Verification items for the finished model (mm, model axes). Face numbers are marked on the shaded views. Round coordinates to 2 decimals unless told otherwise and drop trailing zeros. Write each loop counter-clockwise with the first axis right and the second up, starting at its lowest first coordinate (ties: lowest second). Pieces come first, ordered by that corner, then holes. Notation, with made-up numbers: M 3,-31 L 23,-31 A23 cw 23,8 Z; hole C 22,21.5 d1. An arc over 180 degrees is marked long. One line per question, with ' | ' between items. Start each with the question number.
Q1. Cross-section at A-A (y = 0). Record the boundary of the cut face in (x, z), then the cut area to 3 significant figures.
Q2. Release check for a two-part mould opening along Y. For the marked faces 1, 2 and 3 record: released by +Y, released by -Y, zero draft, split by the parting line, or undercut.
Q3. Thickness scan on line 1 along X through (y, z) = (40.5, 35); line 2 along Y through (x, z) = (-33.5, 27.5); line 3 along Y through (x, z) = (-32.5, 31). Record the ranges inside material, lowest first. Write a range as from..to.
Q4. Cross-section at D-D (x = 40). Record the boundary of the cut face in (y, z), then the cut area to 3 significant figures.
Q5. Gauge pin test, flat ends, axial feed: pin 1 (5 mm diameter, centred on x = 40.5, z = 32.5, fed in from +Y); pin 2 (10 mm diameter, centred on y = 19.5, z = 19.5, fed in from -X); pin 3 (3 mm diameter, centred on x = 9, y = -47.5, fed in from +Z); pin 4 (6 mm diameter, centred on y = -35.5, z = 6.5, fed in from +X). Record the tip position at first contact, or that the pin passes through.
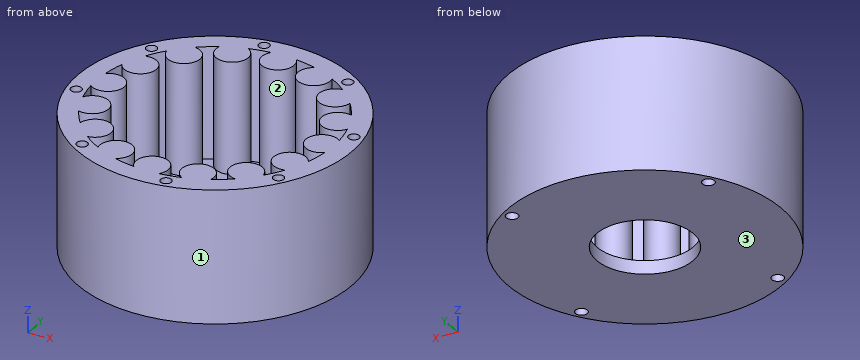
from build123d import *

# Parameters (mm, degrees)
SKETCH1_R           = 44
VOLUMEEXTRUDE_DEPTH = 8
SKETCH2_R           = 51
SKETCH2_R_2         = 44
LIPEXTRUDE_DEPTH    = 49.5
SKETCH4_R           = 18
SHAFT_HOLE_DEPTH    = 8
SKETCH6_R           = 2
BOLTHOLES_DEPTH     = 6
SKETCH7_R           = 6
BOSS_EXTRUDE1_DEPTH = 41.5
SKETCH9_R           = 2.25
CUT_EXTRUDE2_DEPTH  = 6
SKETCH11_R          = 23.6
CUT_EXTRUDE3_DEPTH  = 3


with BuildPart() as part:
    # Sketch1 → VolumeExtrude (new body)
    with BuildSketch(Plane.XY):
        Circle(SKETCH1_R)
    extrude(amount=VOLUMEEXTRUDE_DEPTH)

    # Sketch2 → LipExtrude (add)
    with BuildSketch(Plane(origin=(0, 0, 0), x_dir=(-1, 0, 0), z_dir=(0, 0, -1))):
        Circle(SKETCH2_R)
        Circle(SKETCH2_R_2, mode=Mode.SUBTRACT)
    extrude(amount=-LIPEXTRUDE_DEPTH)

    # Sketch4 → Shaft Hole (cut)
    with BuildSketch(Plane.XY.offset(8)):
        Circle(SKETCH4_R)
    extrude(amount=-SHAFT_HOLE_DEPTH, mode=Mode.SUBTRACT)

    # Sketch6 → BoltHoles (cut)
    with BuildSketch(Plane.XY.offset(49.5)):
        with Locations((-9.06342728, 46.627291214)):
            Circle(SKETCH6_R)
        with Locations((26.561662915, 39.379284696)):
            Circle(SKETCH6_R)
        with Locations((46.627291214, 9.06342728)):
            Circle(SKETCH6_R)
        with Locations((39.379284696, -26.561662915)):
            Circle(SKETCH6_R)
        with Locations((9.06342728, -46.627291214)):
            Circle(SKETCH6_R)
        with Locations((-26.561662915, -39.379284696)):
            Circle(SKETCH6_R)
        with Locations((-46.627291214, -9.06342728)):
            Circle(SKETCH6_R)
        with Locations((-39.379284696, 26.561662915)):
            Circle(SKETCH6_R)
    extrude(amount=-BOLTHOLES_DEPTH, mode=Mode.SUBTRACT)

    # Sketch7 → Boss-Extrude1 (add)
    with BuildSketch(Plane.XY.offset(8)):
        with Locations((0, 40)):
            Circle(SKETCH7_R)
        with Locations((15.307337295, 36.9551813)):
            Circle(SKETCH7_R)
        with Locations((28.284271247, 28.284271247)):
            Circle(SKETCH7_R)
        with Locations((36.9551813, 15.307337295)):
            Circle(SKETCH7_R)
        with Locations((40, 0)):
            Circle(SKETCH7_R)
        with Locations((36.9551813, -15.307337295)):
            Circle(SKETCH7_R)
        with Locations((28.284271247, -28.284271247)):
            Circle(SKETCH7_R)
        with Locations((15.307337295, -36.9551813)):
            Circle(SKETCH7_R)
        with Locations((0, -40)):
            Circle(SKETCH7_R)
        with Locations((-15.307337295, -36.9551813)):
            Circle(SKETCH7_R)
        with Locations((-28.284271247, -28.284271247)):
            Circle(SKETCH7_R)
        with Locations((-36.9551813, -15.307337295)):
            Circle(SKETCH7_R)
        with Locations((-40, 0)):
            Circle(SKETCH7_R)
        with Locations((-36.9551813, 15.307337295)):
            Circle(SKETCH7_R)
        with Locations((-28.284271247, 28.284271247)):
            Circle(SKETCH7_R)
        with Locations((-15.307337295, 36.9551813)):
            Circle(SKETCH7_R)
    extrude(amount=BOSS_EXTRUDE1_DEPTH)

    # Sketch9 → Cut-Extrude2 (cut)
    with BuildSketch(Plane(origin=(0, 0, 0), x_dir=(-1, 0, 0), z_dir=(0, 0, -1))):
        with Locations((-26.561662915, 39.379284696)):
            Circle(SKETCH9_R)
        with Locations((39.379284696, 26.561662915)):
            Circle(SKETCH9_R)
        with Locations((26.561662915, -39.379284696)):
            Circle(SKETCH9_R)
        with Locations((-39.379284696, -26.561662915)):
            Circle(SKETCH9_R)
    extrude(amount=-CUT_EXTRUDE2_DEPTH, mode=Mode.SUBTRACT)

    # Sketch11 → Cut-Extrude3 (cut)
    with BuildSketch(Plane.XY.offset(8)):
        Circle(SKETCH11_R)
    extrude(amount=-CUT_EXTRUDE3_DEPTH, mode=Mode.SUBTRACT)


solid = part.part
Determined:
1) outline: M -51,0 L -18,0 L -18,5 L -23.6,5 L -23.6,8 L -34,8 L -34,49.5 L -51,49.5 Z; M 18,0 L 51,0 L 51,49.5 L 34,49.5 L 34,8 L 23.6,8 L 23.6,5 L 18,5 Z | area: 1,910 mm²
2) face 1: split by the parting line | face 2: undercut | face 3: zero draft
3) line 1: x = -31..-10.47, -5.98..5.98, 10.47..31 | line 2: y = -38.45..-25.32, -20.21..-10.4, 10.4..20.21, 25.32..38.45 | line 3: y = -39.3..-24.01, -19.33..-11.29, 11.29..19.33, 24.01..39.3
4) outline: M -31.64,0 L -28.72,0 L -28.72,6 L -24.4,6 L -24.4,0 L 31.64,0 L 31.64,49.5 L 10.14,49.5 L 10.14,8 L 6,8 L 6,49.5 L -6,49.5 L -6,8 L -10.14,8 L -10.14,49.5 L -24.66,49.5 L -24.66,43.5 L -28.46,43.5 L -28.46,49.5 L -31.64,49.5 Z | area: 2,740 mm²
5) pin 1: stops at y = 34.01 | pin 2: stops at x = -48.9 | pin 3: stops at z = 49.5 | pin 4: stops at x = 39.3
